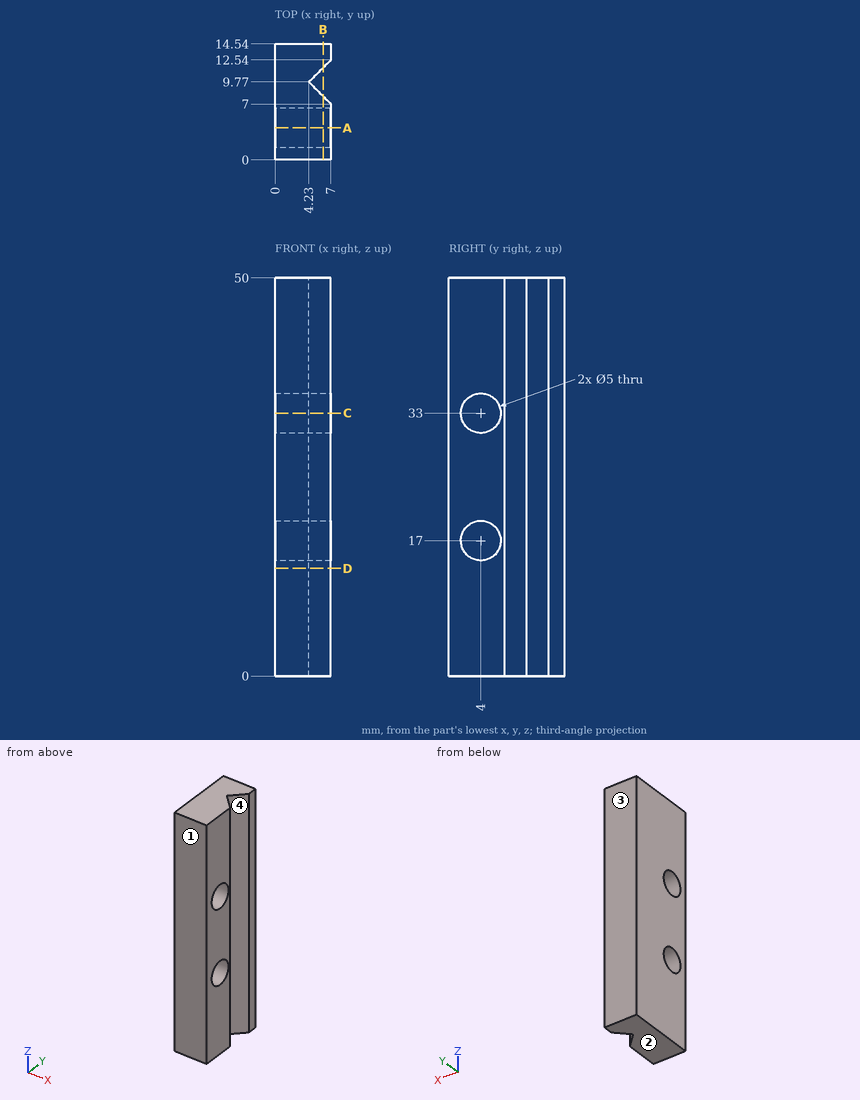
Answer from the drawing. Dimensions are ordinates in mm from the lowest x, y and z of the part. Coordinates: 2 decimals unless noted, no trailing zeros. Write each loop counter-clockwise with the first axis right and the second up, starting at its lowest first coordinate (ties: lowest second). Pieces come first, ordered by that corner, then holes. Notation, with made-up numbers: M 32.25,66.25 L 83.25,66.25 A16 cw 83.25,84.25 Z; hole C 4.5,44.25 d5. An arc over 180 degrees is marked long. Put each result on its own line as item: value. Start each with the question number.
1. For a pull along Y with two mould halves and no side action, classify the marked faces 1, 2, 3 and 4 as pulls with the +Y half, pulls with the -Y half, needs draft (parallel to the pull), parting line crosses it, or undercut.
2. A cutting plane is placed at A-A on y = 4. Write down the section's boundary in (x, z).
3. A cutting plane is placed at C-C on z = 33. Write down the section's boundary in (x, y).
4. A cutting plane is placed at D-D on z = 13.5. Write down the section's boundary in (x, y).
5. Consider line 1 (Z direction, x = 1.5, y = 4.75); line 2 (Z direction, x = 0.5, y = 5.25); line 3 (Y direction, x = 2.75, z = 33). Determine where each line is inside the solid, lowest interval first. Write a range as from..to.
6. A cutting plane is placed at B-B on x = 6. Write down the section's boundary in (y, z), then the cut area to 3 significant figures.
Resolved:
1. face 1: pulls with the -Y half
1. face 2: needs draft
1. face 3: pulls with the +Y half
1. face 4: undercut
2. outline: M 0,0 L 7,0 L 7,14.5 L 0,14.5 Z; M 0,19.5 L 7,19.5 L 7,30.5 L 0,30.5 Z; M 0,35.5 L 7,35.5 L 7,50 L 0,50 Z
3. outline: M 0,0 L 7,0 L 7,1.5 L 0,1.5 Z; M 0,6.5 L 7,6.5 L 7,7 L 4.23,9.77 L 7,12.54 L 7,14.54 L 0,14.54 Z
4. outline: M 0,0 L 7,0 L 7,7 L 4.23,9.77 L 7,12.54 L 7,14.54 L 0,14.54 Z
5. line 1: z = 0..14.62, 19.38..30.62, 35.38..50
5. line 2: z = 0..14.83, 19.17..30.83, 35.17..50
5. line 3: y = 0..1.5, 6.5..14.54
6. outline: M 0,0 L 8,0 L 8,50 L 0,50 Z; M 11.54,0 L 14.54,0 L 14.54,50 L 11.54,50 Z; hole C 4,17 d5; hole C 4,33 d5
6. area: 511 mm2
